from build123d import *

# Parameters (mm, degrees)
SKETCH006_R  = 1.6
PAD007_DEPTH = 1.5
SKETCH_W     = 78
SKETCH_H     = 1.5
PAD008_DEPTH = 17
POCKET_DEPTH = 1.501
FILLET_R     = 4


with BuildPart() as part:
    # Sketch006 → Pad007 (new body)
    with BuildSketch(Plane.XY):
        with BuildLine():
            Line((-35, 21.5), (35, 21.5))
            ThreePointArc((39, 17.5), (37.828427, 20.328427), (35, 21.5))
            Line((39, -21.5), (39, 17.5))
            Line((-39, -21.5), (39, -21.5))
            Line((-39, 17.5), (-39, -21.5))
            ThreePointArc((-35, 21.5), (-37.828427, 20.328427), (-39, 17.5))
        make_face()
        with Locations((-35, -17.5)):
            Circle(SKETCH006_R, mode=Mode.SUBTRACT)
        with Locations((35, 17.5)):
            Circle(SKETCH006_R, mode=Mode.SUBTRACT)
        with Locations((35, -17.5)):
            Circle(SKETCH006_R, mode=Mode.SUBTRACT)
        with Locations((-35, 17.5)):
            Circle(SKETCH006_R, mode=Mode.SUBTRACT)
    extrude(amount=PAD007_DEPTH)

    # Sketch → Pad008 (join)
    with BuildSketch(Plane.XY):
        with Locations((0, -20.75)):
            Rectangle(SKETCH_W, SKETCH_H)
    extrude(amount=-PAD008_DEPTH)

    # Sketch012 (on Face11 of Pad008) → Pocket (cut, through all)
    with BuildSketch(Plane(origin=(0, -20, 0), x_dir=(-1, 0, 0), z_dir=(0, 1, 0))):
        with BuildLine():
            ThreePointArc((-24, -8.4), (-25.6, -10), (-24, -11.6))
            Line((-24, -11.6), (-14, -11.6))
            ThreePointArc((-14, -11.6), (-12.4, -10), (-14, -8.4))
            Line((-14, -8.4), (-24, -8.4))
        make_face()
        with BuildLine():
            ThreePointArc((24, -11.6), (25.6, -10), (24, -8.4))
            Line((14, -8.4), (24, -8.4))
            ThreePointArc((14, -8.4), (12.4, -10), (14, -11.6))
            Line((24, -11.6), (14, -11.6))
        make_face()
    extrude(amount=-POCKET_DEPTH, mode=Mode.SUBTRACT)

    # Fillet
    fillet_edges = [part.edges().sort_by_distance(p)[0] for p in [
        (-39, -20.75, -17),
        (39, -20.75, -17),
    ]]
    fillet(fillet_edges, radius=FILLET_R)


with BuildPart() as part_1:
    # Body001 placement: moved
    add(part.part.moved(Location((0, 0, 65.5))))


solid = part_1.part
Can you work these out from the model? Positions are in its coordinate system, mm. A direction names the side the tool comes from. Round coordinates to 2 decimals unless told otherwise and drop trailing zeros. Loops run counter-clockwise (first coordinate to the right, second up) from the corner with the lowest first, then second, coordinate; pieces in that order, holes last. Notation, with made-up numbers: (-14, 42.5) - (32, 42.5) arc R20 ccw to (32, 75.5) - close; hole circle Ø10 at (67.5, -13.5). An arc over 180 degrees is marked (long way). Use CSV: the item, a comma, the result in double quotes. Start each with the question number.
1) If we section it at A-A on x = 22.5: Write out the boundary of the cut face in (y, z), plus the area to 3 significant figures.
2) If we section it at B-B on z = 55: Write out the boundary of the cut face in (x, y).
3) Please list where these lines run through material, in increasing order: probe 1 along Y at (x, z) = (-35, 66.4); probe 2 along Z at (x, y) = (34.5, 6.5); probe 3 along Y at (x, z) = (-31.5, 62.5). Write a range as [from, to].
4) For pin 1 Ø5 at (x, y) = (-26.5, -6) entering from -Z, with a flat end and sliding along its axis, tell me the tip position at first contact or that it passes through.
5) For faces 4 (the flat face through (-19, -21, 57.1)), 5 (the flat face through (1, 1, 65.5)), 6 (the flat face through (-39, -6, 66)), which set-ups out of +Z, -Z, +X, -X, +Y, -Y let a thin tool reach every point of the face, with its end or its side?
6) If we section it at C-C on y = 3: Write out the boundary of the cut face in (x, z).
7) If we section it at D-D on x = 3: Write out the boundary of the cut face in (y, z), plus the area to 3 significant figures.
8) We'd pull the mould along X, two halves only. Please class faces 1 (the flat face through (-1, -21.5, 58)), 2 (the cylindrical face through (37.797, -20.74, 49.641)), 3 (the cylindrical face through (33.82, 18.58, 66.24)): released by +X, released by -X, zero draft, split by the parting line, or undercut.
Geometry results:
1,outline,"(-21.5, 48.5) - (-20, 48.5) - (-20, 53.9) - (-21.5, 53.9) - close; (-21.5, 57.1) - (-20, 57.1) - (-20, 65.5) - (21.5, 65.5) - (21.5, 67) - (-21.5, 67) - close"
1,area,"85.2 mm2"
2,outline,"(-39, -21.5) - (-25.52, -21.5) - (-25.52, -20) - (-39, -20) - close; (-12.48, -21.5) - (12.48, -21.5) - (12.48, -20) - (-12.48, -20) - close; (25.52, -21.5) - (39, -21.5) - (39, -20) - (25.52, -20) - close"
3,probe 1,"y = [-21.5, -19.1], [-15.9, 15.9], [19.1, 21.5]"
3,probe 2,"z = [65.5, 67]"
3,probe 3,"y = [-21.5, -20]"
4,pin 1,"stops at z = 65.5"
5,face 4,"+Y, -Y"
5,face 5,"-Z, +X, -X, +Y"
5,face 6,"+Z, -Z, -X, +Y, -Y"
6,outline,"(-39, 65.5) - (39, 65.5) - (39, 67) - (-39, 67) - close"
7,outline,"(-21.5, 48.5) - (-20, 48.5) - (-20, 65.5) - (21.5, 65.5) - (21.5, 67) - (-21.5, 67) - close"
7,area,"90.0 mm2"
8,face 1,"zero draft"
8,face 2,"released by +X"
8,face 3,"undercut"
